Autodesk Inventor part; units mm, degrees
ref_plane "YZ Plane" through (0, 0, 0) normal (1, 0, 0) x (0, 1, 0)
ref_plane "XZ Plane" through (0, 0, 0) normal (0, 1, 0) x (-1, 0, 0)
ref_plane "XY Plane" through (0, 0, 0) normal (0, 0, 1) x (1, 0, 0)
sketch "Эскиз1" plane through (0, 0, 0) normal (0, 0, 1) x (1, 0, 0)
  line L0 (-26.3955, 0) -> (-26.3955, 30)
  line L1 (168.6045, 0) -> (168.6045, 30)
  circle A0 centre (161.1045, 7.5) radius 2
  circle A1 centre (-18.8955, 7.5) radius 2
  line L2 (-26.3955, 60.0004) -> (-30.3955, 60.0004)
  line L3 (172.6045, 60.0004) -> (168.6045, 60.0004)
  line L4 (-26.3955, 60.0004) -> (168.6045, 60.0004)
  line L5 (168.6045, 60.0004) -> (168.6045, 0)
  line L6 (168.6045, 0) -> (-26.3955, 0)
  line L7 (-26.3955, 0) -> (-26.3955, 60.0004)
  point P0 (0, 0)
extrude "Выдавливание1" add sketch "Эскиз1" along normal blind 4
thicken "Толщина1" operation add thickness 4 both sides no extend neighbours yes toward (1, 0, 0) faces at (168.6045, 10, 1.3333)
thicken "Толщина2" operation add thickness 4 both sides no extend neighbours yes toward (-1, 0, 0) faces at (-26.3955, 40.0003, 2.6667)
sketch "Эскиз2" plane through (0, 0, 4) normal (0, 0, 1) x (1, 0, 0)
  line L0 (172.6045, 60.0004) -> (-30.3955, 60.0004)
  line L1 (-30.3955, 60.0004) -> (-26.3955, 60.0004)
  line L2 (-26.3955, 60.0004) -> (-26.3955, 48.0004)
  line L3 (-26.3955, 48.0004) -> (-30.3955, 48.0004)
  line L4 (-30.3955, 48.0004) -> (-30.3955, 60.0004)
  line L5 (172.6045, 60.0004) -> (168.6045, 60.0004)
  line L6 (168.6045, 60.0004) -> (168.6045, 48.0004)
  line L7 (168.6045, 48.0004) -> (172.6045, 48.0004)
  line L8 (172.6045, 48.0004) -> (172.6045, 60.0004)
  point P0 (0, 0)
  dimension "d6" = 4
  dimension "d7" = 12
  dimension "d8" = 4
  dimension "d9" = 12
extrude "Выдавливание2" cut sketch "Эскиз2" against normal blind 4
pattern_linear "Прямоуг.массив1" count 3 spacing 24 along (0, -1, 0) of "Выдавливание2"
thicken "Толщина3" operation add thickness 4 both sides no extend neighbours yes toward (1, 0, 0) faces at (-30.3955, 0.0003, 1.3333) (-29.0622, 0.0004, 2.6667)
thicken "Толщина4" operation add thickness 4 both sides no extend neighbours yes toward (-1, 0, 0) faces at (172.6045, 0.0001, 1.3333) (169.9378, 0.0004, 2.6667)
properties part number "KB33-046-004-014 - Лицевая вертикальня пластина" material "Пластик ПЭТ"
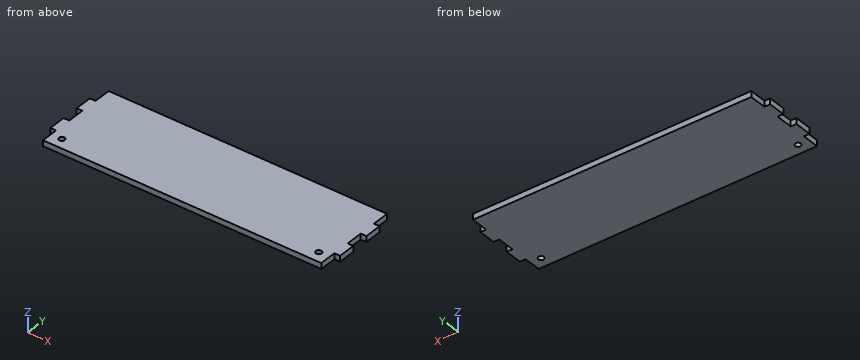
The listing builds one solid part. Answer for the finished solid, in the listing's coordinates (mm). Coordinates: 2 decimals unless noted, no trailing zeros. Write each loop counter-clockwise with the first axis right and the second up, starting at its lowest first coordinate (ties: lowest second). Pieces come first, ordered by that corner, then holes. Notation, with made-up numbers: (15, -4) - (35, -4) arc R5 cw to (35, 0) - close; hole circle Ø1 at (19.25, 7). An arc over 180 degrees is marked (long way). Return JSON: item names as keys, results as strings.
1. Each of these flat-tipped pins is pushed along its axis until it touches: pin 1 Ø1.2 at (x, z) = (171.5, 2.5) entering from -Y; pin 2 Ø1.2 at (x, z) = (171.5, 1.5) entering from +Y; pin 3 Ø2 at (y, z) = (56, 1.5) entering from -X. Where does it stop, or does it pass through?
Final values:
{"pin 1": "y = 12", "pin 2": "y = 48", "pin 3": "x = -26.4"}
2. The part is cut by section B-B on y = 7.5. Determine the outline of the cut face in (x, z).
Final values:
{"outline": "(-26.4, 0) - (-20.9, 0) - (-20.9, 4) - (-26.4, 4) - close; (-16.9, 0) - (159.1, 0) - (159.1, 4) - (-16.9, 4) - close; (163.1, 0) - (168.6, 0) - (168.6, 4) - (163.1, 4) - close"}
3. The part is cut by section A-A on z = 1.75. Determine the outline of the cut face in (x, y), then the cut area to 3 significant figures.
Final values:
{"outline": "(-30.4, 12) - (-26.4, 12) - (-26.4, 0) - (168.6, 0) - (168.6, 12) - (172.6, 12) - (172.6, 24) - (168.6, 24) - (168.6, 36) - (172.6, 36) - (172.6, 48) - (168.6, 48) - (168.6, 60) - (-26.4, 60) - (-26.4, 48) - (-30.4, 48) - (-30.4, 36) - (-26.4, 36) - (-26.4, 24) - (-30.4, 24) - close; hole circle Ø4 at (-18.9, 7.5); hole circle Ø4 at (161.1, 7.5)", "area": "11,900 mm^2"}
4. Consider line 1 along X through (y, z) = (7.5, 1.2); line 2 along X through (y, z) = (27.5, 2.45). Determine where each line is inside the solid, lowest interval first.
Final values:
{"line 1": "-26.4 to -20.9, -16.9 to 159.1, 163.1 to 168.6", "line 2": "-26.4 to 168.6"}
5. The part is cut by section C-C on y = 27.5. Determine the outline of the cut face in (x, z).
Final values:
{"outline": "(-26.4, 0) - (168.6, 0) - (168.6, 4) - (-26.4, 4) - close"}
